Verification items for the finished model (mm, model axes). A direction names the side the tool comes from. Coordinates: 2 decimals unless noted, no trailing zeros. Write each loop counter-clockwise with the first axis right and the second up, starting at its lowest first coordinate (ties: lowest second). Pieces come first, ordered by that corner, then holes. Notation, with made-up numbers: M 42,-22.75 L 79,-22.75 A33 ccw 79,15.25 Z; hole C 63,-13.5 d2. An arc over 180 degrees is marked long. Answer in a Markdown table with one row per item.
from build123d import *

# Parameters (mm, degrees)
F0_W      = 100
F0_H      = 50
F1_DEPTH  = 50
F2_T      = -3
F3_W      = 7.189277
F3_H      = 13.505568
F4_DEPTH  = 3
F3_W_2    = 9.575039
F3_H_2    = 10.380805
F5_DEPTH  = 3
F6_R      = 2.5
F7_DEPTH  = 5
F6_R_2    = 2.717487
F8_DEPTH  = 5
F6_R_3    = 2.762406
F9_DEPTH  = 5
F6_R_4    = 2.52466
F10_DEPTH = 5


with BuildPart() as f1:
    # F0 (on Front) → F1 (new body)
    with BuildSketch(Plane.XZ):
        with Locations((-9.887868, -10.982526)):
            Rectangle(F0_W, F0_H)
    extrude(amount=F1_DEPTH)

    # F2
    f2_openings = [f1.faces().sort_by_distance(p)[0] for p in [
        (-9.887868, -50, -10.982526),
    ]]
    offset(amount=F2_T, openings=f2_openings)

    # F3 (on face) → F4 (cut)
    with BuildSketch(Plane.YZ.offset(40.112132)):
        with Locations((-11.745577, -3.117744)):
            Rectangle(F3_W, F3_H)
    extrude(amount=-F4_DEPTH, mode=Mode.SUBTRACT)

    # F3 (on face) → F5 (cut)
    with BuildSketch(Plane.YZ.offset(40.112132)):
        with Locations((-30.345603, -21.830169)):
            Rectangle(F3_W_2, F3_H_2)
    extrude(amount=-F5_DEPTH, mode=Mode.SUBTRACT)

    # F6 (on face) → F7 (join)
    with BuildSketch(Plane.XZ.offset(3)):
        with Locations((21.496529, 2.875064)):
            Circle(F6_R)
    extrude(amount=F7_DEPTH)

    # F6 (on face) → F8 (join)
    with BuildSketch(Plane.XZ.offset(3)):
        with Locations((21.496529, -18.16091)):
            Circle(F6_R_2)
    extrude(amount=F8_DEPTH)

    # F6 (on face) → F9 (join)
    with BuildSketch(Plane.XZ.offset(3)):
        with Locations((-15.370856, -18.16091)):
            Circle(F6_R_3)
    extrude(amount=F9_DEPTH)

    # F6 (on face) → F10 (join)
    with BuildSketch(Plane.XZ.offset(3)):
        with Locations((-15.370856, 2.875064)):
            Circle(F6_R_4)
    extrude(amount=F10_DEPTH)


solid = f1.part
1) Sectioned sample at B-B (y = -42). Record the cut outline in (x, z), then the cut area to 3 significant figures.
Response values:
| item | result |
|---|---|
| outline | M -59.89,-35.98 L 40.11,-35.98 L 40.11,14.02 L -59.89,14.02 Z; hole M -56.89,-32.98 L 37.11,-32.98 L 37.11,11.02 L -56.89,11.02 Z |
| area | 864 mm² |
2) Depth check by flat-ended pin: pin 1 (12 mm diameter, centred on x = -45.5, z = -17, fed in from -Y); pin 2 (4.5 mm diameter, centred on x = -14.5, z = -18, fed in from -Y). Enter the tip coordinate at first touch or a pass-through.
Response values:
| item | result |
|---|---|
| pin 1 | stops at y = -3 |
| pin 2 | stops at y = -8 |
3) Sectioned sample at D-D (y = -13). Record the cut outline in (x, z), then the cut area to 3 significant figures.
Response values:
| item | result |
|---|---|
| outline | M -59.89,-35.98 L 40.11,-35.98 L 40.11,-9.87 L 37.11,-9.87 L 37.11,-32.98 L -56.89,-32.98 L -56.89,11.02 L 37.11,11.02 L 37.11,3.64 L 40.11,3.64 L 40.11,14.02 L -59.89,14.02 Z |
| area | 823 mm² |
4) Tool access check on faces 4 (the face through (-11, -26, 11.017)), 5 (the face through (39, -30, -27.021)), 6 (the face through (-59.888, -25, -11)). Record the directions out of +Z, -Z, +X, -X, +Y, -Y that give a thin tool (end or side, any length) a straight path to the whole face; none if there is none.
Response values:
| item | result |
|---|---|
| face 4 | -Y |
| face 5 | +X |
| face 6 | +Z, -Z, -X, +Y, -Y |
5) Sectioned sample at C-C (x = -35.5). Record the cut outline in (y, z), then the cut area to 3 significant figures.
Response values:
| item | result |
|---|---|
| outline | M -50,-35.98 L 0,-35.98 L 0,14.02 L -50,14.02 L -50,11.02 L -3,11.02 L -3,-32.98 L -50,-32.98 Z |
| area | 432 mm² |
6) Thickness scan on L1, parallel to Z at x = 5, y = -14; L2, parallel to X at y = -18, z = -24; L3, parallel to Y at x = -22.5, z = -12. Record the ranges inside material, lowest first. Write a range as [from, to].
Response values:
| item | result |
|---|---|
| L1 | z = [-35.98, -32.98], [11.02, 14.02] |
| L2 | x = [-59.89, -56.89], [37.11, 40.11] |
| L3 | y = [-3, 0] |
7) Sectioned sample at A-A (z = -26). Record the cut outline in (x, y), then the cut area to 3 significant figures.
Response values:
| item | result |
|---|---|
| outline | M -59.89,-50 L -56.89,-50 L -56.89,-3 L 37.11,-3 L 37.11,-25.56 L 40.11,-25.56 L 40.11,0 L -59.89,0 Z; M 37.11,-50 L 40.11,-50 L 40.11,-35.13 L 37.11,-35.13 Z |
| area | 553 mm² |
8) Release check for a two-part mould opening along Z. For faces 1 (the face through (40.112, -25, -11)), 2 (the face through (39, -12, 3.635)), 3 (the face through (-11, -25, -35.983)) record: +Z half, -Z half, draft (parallel to the pull), parting line (faces both ways), or undercut.
Response values:
| item | result |
|---|---|
| face 1 | draft |
| face 2 | undercut |
| face 3 | -Z half |
